Part model, mm, in its own coordinate system. Face numbers are marked on the shaded views. Coordinates: 2 decimals unless noted, no trailing zeros. Write each loop counter-clockwise with the first axis right and the second up, starting at its lowest first coordinate (ties: lowest second). Pieces come first, ordered by that corner, then holes. Notation, with made-up numbers: M 52.25,4.5 L 109.25,4.5 A26 ccw 109.25,24.5 Z; hole C -3.75,12.5 d11. An arc over 180 degrees is marked long. Use a Markdown table: item, result. Add a question column.
Q1. Mould opens along X. For the marked faces 1, 2 and 3 say: released by +X, released by -X, zero draft, split by the parting line, or undercut.
Q2. Pin check, flat tips, straight feed: pin 1 Ø1 at (y, z) = (0.5, -9.5) entering from +X; pin 2 Ø8 at (x, z) = (16.5, -22.5) entering from -Y; pin 3 Ø4.5 at (x, z) = (10, -2.5) entering from +Y; pin 4 Ø1.5 at (y, z) = (0.5, 24.5) entering from +X. Stop position of each tip, or through.
Q3. Wall check: L1, parallel to X at y = -0.25, z = -5; L2, parallel to X at y = 3.75, z = 17.5; L3, parallel to Y at x = 6.5, z = 6. Give the ranges that are in metal, low to high. Write a range as from..to.
Q4. Slice it at A-A on y = 0.75. Count the separate pieces of the cut face and the enclosed holes in it, then the cut area to 3 significant figures.
Q5. Slice it at B-B on y = 6. Write the cut outline in (x, z), then the cut area to 3 significant figures.
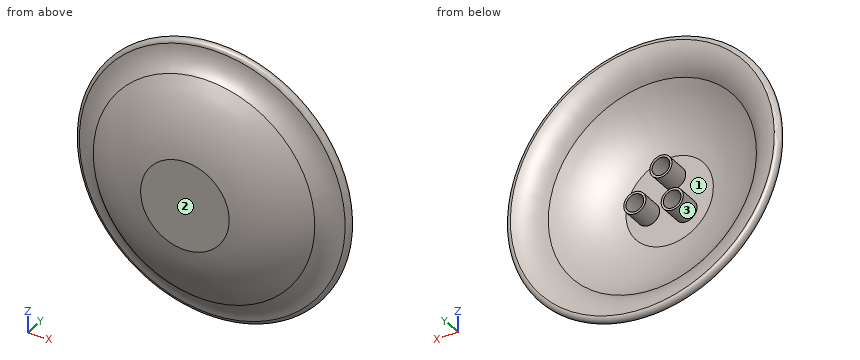
from build123d import *

# Parameters (mm, degrees)
SKETCH2_R           = 2.5
SKETCH2_R_2         = 2
BOSS_EXTRUDE2_DEPTH = 5


with BuildPart() as part:
    # Sketch1 → Revolve1 (revolve)
    with BuildSketch(Plane.XY, mode=Mode.PRIVATE) as revolve1_sk:
        with BuildLine():
            Line((3.119266055, -4.816513761), (13.119266055, -4.816513761))
            Line((13.119266055, -4.816513761), (13.119266055, -2.816513761))
            Line((13.119266055, -2.816513761), (3.257916771, -2.816513761))
            ThreePointArc((3.257916771, -2.816513761), (-4.025816821, -0.658797724), (-10.372175668, 3.516396035))
            ThreePointArc((-10.372175668, 3.516396035), (-13.131249362, 6.018603225), (-16.672681055, 7.172635302))
            ThreePointArc((-16.672681055, 7.172635302), (-17.771282031, 6.282087215), (-16.880733945, 5.183486239))
            ThreePointArc((-16.880733945, 5.183486239), (-14.048292509, 4.237555299), (-11.880733945, 2.183486239))
            ThreePointArc((-11.880733945, 2.183486239), (-4.911005239, -2.452809391), (3.119266055, -4.816513761))
        make_face()
    revolve(revolve1_sk.sketch.rotate(Axis((13.119266055, -2.816513761, 0), (0, -1, 0)), 270), axis=Axis((13.119266055, -2.816513761, 0), (0, -1, 0)))

    # Sketch2 → Boss-Extrude2 (add)
    # profile 1 of 3: a face of its own
    with BuildSketch(Plane(origin=(0, -2.816513761, 0), x_dir=(1, 0, 0), z_dir=(0, 1, 0))):
        with Locations(Location((9.455762685, 3.402755216, 0), (0, 0, 270))):
            Circle(SKETCH2_R)
        with Locations(Location((9.455762685, 3.402755216, 0), (0, 0, 270))):
            Circle(SKETCH2_R_2, mode=Mode.SUBTRACT)
    # profile 2 of 3: a face of its own
    with BuildSketch(Plane(origin=(0, -2.816513761, 0), x_dir=(1, 0, 0), z_dir=(0, 1, 0))):
        with Locations(Location((17.8978902, 1.471309377, 0), (0, 0, 270))):
            Circle(SKETCH2_R)
        with Locations(Location((17.8978902, 1.471309377, 0), (0, 0, 270))):
            Circle(SKETCH2_R_2, mode=Mode.SUBTRACT)
    # profile 3 of 3: a face of its own
    with BuildSketch(Plane(origin=(0, -2.816513761, 0), x_dir=(1, 0, 0), z_dir=(0, 1, 0))):
        with Locations(Location((12.00414528, -4.874064593, 0), (0, 0, 270))):
            Circle(SKETCH2_R)
        with Locations(Location((12.00414528, -4.874064593, 0), (0, 0, 270))):
            Circle(SKETCH2_R_2, mode=Mode.SUBTRACT)
    extrude(amount=BOSS_EXTRUDE2_DEPTH)


solid = part.part
Recorded:
| question | item | result |
|---|---|---|
| 1 | face 1 | undercut |
| 1 | face 2 | zero draft |
| 1 | face 3 | undercut |
| 2 | pin 1 | x = 34.77 |
| 2 | pin 2 | y = -2.1 |
| 2 | pin 3 | y = 2.18 |
| 2 | pin 4 | through |
| 3 | L1 | -8.21..-4.16, 7.53..8.25, 10.66..11.38, 30.4..34.45 |
| 3 | L2 | -6.73..-2.81, 29.05..32.96 |
| 3 | L3 | -4.82..-2.82 |
| 4 | separate pieces | 4 |
| 4 | enclosed holes | 4 |
| 4 | area | 497 mm² |
| 5 | outline | C 13.12,0 d61.76; hole C 13.12,0 d52.44 |
| 5 | area | 836 mm² |
